```python
from build123d import *

# Parameters (mm, degrees)
SKETCH_1_W          = 375.14
SKETCH_1_H          = 215.14
EXTRUDE_1_DEPTH     = 250
SHELL_1_T           = -10
SKETCH_5_R          = 12.5
CUT_EXTRUDE_1_DEPTH = 10
SKETCH_6_W          = 214
SKETCH_6_H          = 54
CUT_EXTRUDE_2_DEPTH = 10


with BuildPart() as part:
    # 草图1 → 凸台-拉伸1 (new body)
    with BuildSketch(Plane(origin=(0, 0, 0), x_dir=(1, 0, 0), z_dir=(0, 1, 0))):
        Rectangle(SKETCH_1_W, SKETCH_1_H)
    extrude(amount=EXTRUDE_1_DEPTH)

    # 草图4 → section 1 of loft_1
    with BuildSketch(Plane(origin=(0, -130, 0), x_dir=(1, 0, 0), z_dir=(0, 1, 0)), mode=Mode.PRIVATE) as loft_1_s1:
        with BuildLine():
            Line((-112, 32), (112, 32))
            Line((112, 32), (112, -32))
            Line((112, -32), (-112, -32))
            Line((-112, -32), (-112, 32))
        make_face()
    # loft from a face of the part (loft_1)
    loft([part.faces().sort_by_distance((0, 0, 0))[0], loft_1_s1.sketch])

    # 抽壳1
    shell_1_openings = [part.faces().sort_by_distance(p)[0] for p in [
        (0, 250, 0),
    ]]
    offset(amount=SHELL_1_T, openings=shell_1_openings, kind=Kind.INTERSECTION)

    # 草图5 → 切除-拉伸1 (cut)
    with BuildSketch(Plane.XY.offset(107.57)):
        with Locations((0, 177)):
            Circle(SKETCH_5_R)
    extrude(amount=-CUT_EXTRUDE_1_DEPTH, mode=Mode.SUBTRACT)

    # 草图6 → 切除-拉伸2 (cut)
    with BuildSketch(Plane.XZ.offset(130)):
        Rectangle(SKETCH_6_W, SKETCH_6_H)
    extrude(amount=-CUT_EXTRUDE_2_DEPTH, mode=Mode.SUBTRACT)


solid = part.part
```
Check sheet for the modelled part. Datum: model origin and axes. Units: mm. A direction names the side the tool comes from. Give positions to 0.01 mm unless a question says otherwise; leave off trailing zeros. Order: outer loops, then holes, each group sorted by start corner. A loop starts at its lowest first (then second) coordinate and runs counter-clockwise, first axis right, second up. Notation, with made-up numbers: (-15, -28) -> (43, -28) arc R26 cw to (43, 9) -> close; hole circle Ø9 at (-5, -23.5). An arc over 180 degrees is marked (long way). Return JSON: item names as keys, results as strings.
1. Material ranges on probe 1 along X at (y, z) = (116, -1); probe 2 along Z at (x, y) = (150, 31.5); probe 3 along Y at (x, z) = (0, 102.5), recorded low to high. Write a range as [from, to].
From the geometry:
{"probe 1": "[-187.57, -177.57], [177.57, 187.57]", "probe 2": "[-107.57, -97.57], [97.57, 107.57]", "probe 3": "[-8.72, 164.5], [189.5, 250]"}
2. Set-up check for faces 1 (the flat face through (-1, -125, 27)), 2 (the flat face through (177.57, 125, 1)), 3 (the flat face through (-3, 123, -107.57)): record each of +Z, -Z, +X, -X, +Y, -Y from which the full face is reachable in a straight line by a thin tool's end or side.
From the geometry:
{"face 1": "-Y", "face 2": "+Y", "face 3": "-Z, +X, -X, +Y, -Y"}
3. Go/stop test with flat-tipped pins: P1, Ø8, axis at y = -127, z = -2.5, coming from the -X side; P2, Ø3, axis at x = 139, z = 15, coming from the +Y side; P3, Ø11, axis at x = 36.5, y = -123.5, coming from the +Z side. Record where each tip stops, or that it passes through.
From the geometry:
{"P1": "x = -116.07", "P2": "y = -61.07", "P3": "z = 38.98"}
4. Mould release check, pull along Y, two halves, no side actions. Record for faces 4 (the flat face through (-1, -130, 29)), 5 (the flat face through (-187.57, 123, 2)), 6 (the cylindrical face through (-1.627, 189.394, 102.64)): +Y half, -Y half, draft (parallel to the pull), parting line (faces both ways), or undercut.
From the geometry:
{"face 4": "-Y half", "face 5": "draft", "face 6": "undercut"}
5. Cross-section at C-C, the plane x = 0. Count the separate pieces of the cut face and the enclosed holes in it, plus the area to 3 significant figures.
From the geometry:
{"separate pieces": "3", "enclosed holes": "0", "area": "7,690 mm^2"}
6. Cross-section at B-B, the plane y = 177. Record the cut outline in (x, z), plus the area to 3 significant figures.
From the geometry:
{"outline": "(-187.57, -107.57) -> (187.57, -107.57) -> (187.57, 107.57) -> (12.5, 107.57) -> (12.5, 97.57) -> (177.57, 97.57) -> (177.57, -97.57) -> (-177.57, -97.57) -> (-177.57, 97.57) -> (-12.5, 97.57) -> (-12.5, 107.57) -> (-187.57, 107.57) -> close", "area": "11,200 mm^2"}
7. Cross-section at A-A, the plane y = 46. Record the cut outline in (x, z).
From the geometry:
{"outline": "(-187.57, -107.57) -> (187.57, -107.57) -> (187.57, 107.57) -> (-187.57, 107.57) -> close; hole (-177.57, -97.57) -> (177.57, -97.57) -> (177.57, 97.57) -> (-177.57, 97.57) -> close"}
